Model file for the job. Use its own axes, mm. Face numbers are marked on the shaded views. A direction names the side the tool comes from. Coordinates: 2 decimals unless noted, no trailing zeros. Loops run counter-clockwise (first coordinate to the right, second up) from the corner with the lowest first, then second, coordinate; pieces in that order, holes last.
from build123d import *

# Parameters (mm, degrees)
AUFSATZ_LINEAR_AUSTRAGEN1_DEPTH = 7.5
SCHNITT_LINEAR_AUSTRAGEN1_DEPTH = 10
SKIZZE7_R                       = 2.5
SCHNITT_LINEAR_AUSTRAGEN4_DEPTH = 84.113251049
M4_GEWINDEBOHRUNG1_D            = 3.3
M4_GEWINDEBOHRUNG1_DEPTH        = 7.5
M4_GEWINDEBOHRUNG1_TIP          = 0.991420021
SKIZZE9_OUTSIDE_W               = 26.654
SKIZZE9_OUTSIDE_H               = 99.154
SKIZZE9_OUTSIDE_R               = 1.5
SCHNITT_LINEAR_AUSTRAGEN5_DEPTH = 6
SKIZZE10_OUTSIDE_W              = 26.654
SKIZZE10_OUTSIDE_H              = 99.154
SKIZZE10_OUTSIDE_R              = 1.5
SCHNITT_LINEAR_AUSTRAGEN6_DEPTH = 6


with BuildPart() as part:
    # Skizze1 → Aufsatz-Linear austragen1 (new body)
    with BuildSketch(Plane.XY):
        with BuildLine():
            Line((-8.75, 75), (-3.25, 75))
            ThreePointArc((-3.25, 75), (-0.951902961, 74.048097039), (0, 71.75))
            Line((0, 71.75), (0, 2))
            Line((0, 2), (2, 0))
            Line((2, 0), (10.5, 0))
            Line((10.5, 0), (12.5, 2))
            Line((12.5, 2), (12.5, 71.75))
            ThreePointArc((12.5, 71.75), (13.451902961, 74.048097039), (15.75, 75))
            Line((15.75, 75), (21.25, 75))
            Line((21.25, 75), (21.25, 80))
            Line((21.25, 80), (-8.75, 80))
            Line((-8.75, 80), (-8.75, 75))
        make_face()
    extrude(amount=AUFSATZ_LINEAR_AUSTRAGEN1_DEPTH)

    # Skizze2 → Schnitt-Linear austragen1 (cut)
    with BuildSketch(Plane.XY.offset(7.5)):
        with BuildLine():
            Line((10, 71.25), (10, 13.75))
            ThreePointArc((10, 13.75), (6.25, 10), (2.5, 13.75))
            Line((2.5, 13.75), (2.5, 71.25))
            ThreePointArc((2.5, 71.25), (6.25, 75), (10, 71.25))
        make_face()
    extrude(amount=-SCHNITT_LINEAR_AUSTRAGEN1_DEPTH, mode=Mode.SUBTRACT)

    # Skizze7 → Schnitt-Linear austragen4 (cut, through all)
    with BuildSketch(Plane(origin=(12.5, 0, 0), x_dir=(0, 0, -1), z_dir=(1, 0, 0))):
        with Locations(Location((-3.75, 6.25, 0), (0, 0, 90))):
            Circle(SKIZZE7_R)
    extrude(amount=-SCHNITT_LINEAR_AUSTRAGEN4_DEPTH, mode=Mode.SUBTRACT)

    # M4 Gewindebohrung1
    with Locations(Plane(origin=(6.25, 0, 3.75), x_dir=(0, 0, -1), z_dir=(0, -1, 0))):
        with Locations((0, 0)):
            Hole(M4_GEWINDEBOHRUNG1_D / 2, depth=M4_GEWINDEBOHRUNG1_DEPTH)
            with Locations((0, 0, -(M4_GEWINDEBOHRUNG1_DEPTH + M4_GEWINDEBOHRUNG1_TIP / 2))):  # 118° drill point
                Cone(0, M4_GEWINDEBOHRUNG1_D / 2, M4_GEWINDEBOHRUNG1_TIP, mode=Mode.SUBTRACT)

    # Skizze9 outside → Schnitt-Linear austragen5 (cut)
    with BuildSketch(Plane(origin=(21.25, 0, 0), x_dir=(0, 0, -1), z_dir=(1, 0, 0))):
        with Locations((-3.75, 40)):
            Rectangle(SKIZZE9_OUTSIDE_W, SKIZZE9_OUTSIDE_H)
        with Locations((-3.75, 77.5)):
            Circle(SKIZZE9_OUTSIDE_R, mode=Mode.SUBTRACT)
    extrude(amount=-SCHNITT_LINEAR_AUSTRAGEN5_DEPTH, mode=Mode.SUBTRACT)

    # Skizze10 outside → Schnitt-Linear austragen6 (cut)
    with BuildSketch(Plane.ZY.offset(8.75)):
        with Locations((3.75, 40)):
            Rectangle(SKIZZE10_OUTSIDE_W, SKIZZE10_OUTSIDE_H)
        with Locations(Location((3.75, 77.5, 0), (0, 0, 180))):
            Circle(SKIZZE10_OUTSIDE_R, mode=Mode.SUBTRACT)
    extrude(amount=-SCHNITT_LINEAR_AUSTRAGEN6_DEPTH, mode=Mode.SUBTRACT)


solid = part.part
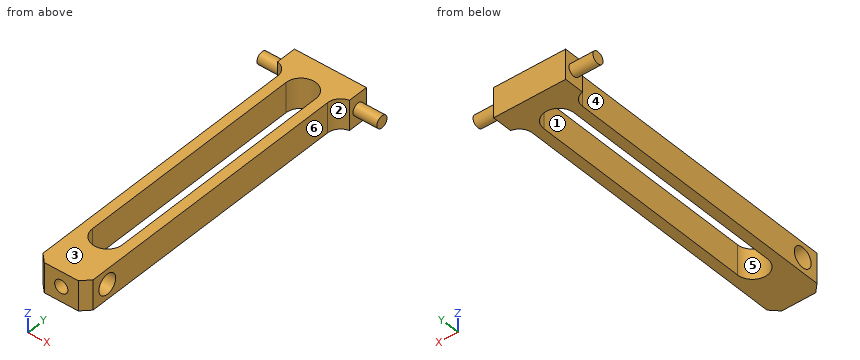
Q1. Drill centre lines: line 1 (X direction, y = 18.5, z = 2); line 2 (Z direction, x = 6.25, y = 3.15); line 3 (Z direction, x = 5.5, y = 6.25). Where is each one in solid material? Low to high.
Answers:
line 1: x = 0 to 2.5, 10 to 12.5
line 2: z = 0 to 2.1, 5.4 to 7.5
line 3: z = 0 to 1.25, 6.25 to 7.5
Q2. Slice it at B-B (z = 3.75). Count the separate pieces of the cut face and the enclosed holes in it, and give its area (3 significant figures).
Answers:
separate pieces: 3
enclosed holes: 1
area: 514 mm2
Q3. Slice it at C-C (x = 6.25). List the corners of the cut face in (y, z), and give its area (3 significant figures).
Answers:
outline: (0, 0) - (10, 0) - (10, 7.5) - (0, 7.5) - (0, 5.4) - (4.37, 5.4) arc R2.5 cw (long way) to (4.37, 2.1) - (0, 2.1) - close; (75, 0) - (80, 0) - (80, 7.5) - (75, 7.5) - close
area: 79.8 mm2
Q4. Slice it at D-D (y = 77.5). List the corners of the cut face in (x, z).
Answers:
outline: (-8.75, 2.25) - (-2.75, 2.25) - (-2.75, 0) - (15.25, 0) - (15.25, 2.25) - (21.25, 2.25) - (21.25, 5.25) - (15.25, 5.25) - (15.25, 7.5) - (-2.75, 7.5) - (-2.75, 5.25) - (-8.75, 5.25) - close
Q5. Mould opens along X. For the marked faces 1, 2 and 3 say: +X half, -X half, draft (parallel to the pull), parting line (faces both ways), or undercut.
Answers:
face 1: undercut
face 2: +X half
face 3: draft
Q6. Flat gauge pins, fed straight in: P1, Ø2, axis at y = 32.5, z = 5, coming from the -X side; P2, Ø4, axis at x = 5, y = 22.5, coming from the +Z side; P3, Ø4, axis at y = 27.5, z = 4.5, coming from the +X side; P4, Ø1.5, axis at y = 72, z = 1, coming from the -X side. Where does each tip first touch, or does it go through?
Answers:
P1: stops at x = 0
P2: passes through
P3: stops at x = 12.5
P4: stops at x = -0.16
Q7. Which spindle directions (+Z, -Z, +X, -X, +Y, -Y) get a long thin tool onto all of the face, cutting with end or side? Do the marked faces 4, 5 and 6. Say none if no direction does.
Answers:
face 4: +Z, -Z, -X, -Y
face 5: +Z, -Z
face 6: +Z, -Z, +X, -Y
Q8. Slice it at A-A (y = 24.5). List the corners of the cut face in (x, z).
Answers:
outline: (0, 0) - (2.5, 0) - (2.5, 7.5) - (0, 7.5) - close; (10, 0) - (12.5, 0) - (12.5, 7.5) - (10, 7.5) - close
